Build history of the part. All positions in model axes, mm. Face numbers are marked on the shaded views. A direction names the side the tool comes from. Round coordinates to 2 decimals unless told otherwise and drop trailing zeros. Write each loop counter-clockwise with the first axis right and the second up, starting at its lowest first coordinate (ties: lowest second). Pieces come first, ordered by that corner, then holes. Notation, with made-up numbers: M -21.5,-37 L -2.5,-37 A27 cw -2.5,-20 Z; hole C 34,-14.75 d9. An arc over 180 degrees is marked long. Write item = value, one per line. Start each with the question number.
Q1. Tool access for the marked faces 4 and 5: list every direction of +Z, -Z, +X, -X, +Y, -Y with a clear straight run to the whole face (end or side of a thin tool).
Q2. Pull direction Y, two halves, no side cores. Call the marked faces 1, 2 and 3: released by +Y, released by -Y, zero draft, split by the parting line, or undercut.
Q3. Probe L1, parallel to X at y = 0.25, z = 2.75; L2, parallel to Z at x = 11.5, y = 0; L3, parallel to Z at x = -1, y = 0.75. List the from-to ranges inside material, lowest first.
Q4. Band-saw the part on A-A on x = 8.5. Write the cut outline in (y, z).
Q5. Drop flat-ended pins along their axis: P1, Ø1, axis at x = 6.5, z = 1.5, coming from the +Y side; P2, Ø1.5, axis at x = 1.5, z = 0.5, coming from the +Y side; P3, Ø0.8, axis at y = -1, z = -1.5, coming from the +X side; P4, Ø0.5, axis at y = -1.5, z = 1.5, coming from the +X side. Give the stop position or say it passes through.
Autodesk Inventor part; units mm, degrees
ref_plane "Work Plane1" through (10.35, 0, 0) normal (0, -0.6335, -0.7737) x (1, 0, 0)
ref_plane "YZ Plane" through (0, 0, 0) normal (1, 0, 0) x (0, 1, 0)
ref_plane "XZ Plane" through (0, 0, 0) normal (0, 1, 0) x (-1, 0, 0)
sketch "Szkic1" plane through (0, 0, 0) normal (0, 0, 1) x (1, 0, 0)
  line L0 (0.0003, 0) -> (20, 0)
  line L1 (20, 0) -> (20, 2)
  line L2 (20, 2) -> (0.7, 2)
  line L3 (0.7, 2) -> (0.2706, 1.8)
  line L4 (0.2706, 1.8) -> (0, 1.8)
  line L5 (0, 1.8) -> (0, 3.5)
  line L6 (0, 3.5) -> (-2.8, 3.5)
  line L7 (-2.8, 3.5) -> (-2.8, 1.975)
  line L8 (-2.8, 1.975) -> (-1.14, 1.975)
  line L9 (-1.14, 1.975) -> (0.0003, 0)
  line L10 (-7.36, 0) -> (24.56, 0)
  line L11 (0, -0.7) -> (0, 4.2)
  line L12 (0.7, 2) -> (0, 2) construction
  dimension "d1" = 19.3
  dimension "d2" = 0.4294
  dimension "d3" = 2.8
  dimension "d4" = 1.66
  dimension "d5" = 60
  dimension "d6" = 4
  dimension "d7" = 3.6
  dimension "d8" = 3.95
  dimension "d9" = 7
  dimension "d20" = 20
revolve "Bryła" add sketch "Szkic1" angle 360 about axis through (0.0003, 0, 0) along (1, 0, 0)
sketch "Szkic2" plane through (-2.8, 0, 0) normal (-1, 0, 0) x (0, 0, 1)
  line L0 (0, -4.9) -> (0, 4.9)
  line L1 (-4.9, 0) -> (4.9, 0)
  circle A0 centre (0, 0) radius 1.975 construction
  circle A1 centre (0, 0) radius 1.425 construction
  line L2 (0, 0) -> (1.7104, 0.9875) construction
  line L3 (0, 0) -> (0.9875, 1.7104) construction
  arc A2 (1.1195, 1.4173) -> (0.6677, 1.6781) centre (0.85, 1.4722) ccw
  arc A3 (1.1195, 1.4173) -> (1.7871, 0.2608) centre (2.1063, 1.2161) ccw
  arc A4 (1.7871, -0.2608) -> (1.7871, 0.2608) centre (1.7, 0) ccw
  arc A5 (1.7871, -0.2608) -> (1.1195, -1.4173) centre (2.1063, -1.2161) ccw
  arc A6 (-0.6677, 1.6781) -> (0.6677, 1.6781) centre (0, 2.4322) ccw
  arc A7 (-0.6677, 1.6781) -> (-1.1195, 1.4173) centre (-0.85, 1.4722) ccw
  arc A8 (-1.7871, 0.2608) -> (-1.1195, 1.4173) centre (-2.1063, 1.2161) ccw
  arc A9 (-1.7871, 0.2608) -> (-1.7871, -0.2608) centre (-1.7, 0) ccw
  arc A10 (-1.1195, -1.4173) -> (-1.7871, -0.2608) centre (-2.1063, -1.2161) ccw
  arc A11 (0.6677, -1.6781) -> (1.1195, -1.4173) centre (0.85, -1.4722) ccw
  arc A12 (0.6677, -1.6781) -> (-0.6677, -1.6781) centre (0, -2.4322) ccw
  arc A13 (-1.1195, -1.4173) -> (-0.6677, -1.6781) centre (-0.85, -1.4722) ccw
  circle A14 centre (0, 0) radius 1.975
  dimension "d34" = 30
  dimension "d35" = 60
  dimension "d36" = 2.85
  dimension "d37" = 3.95
  dimension "d38" = 0.275
extrude "Szczelina" add sketch "Szkic2" against normal blind 1.66 contours A14 A13 A12 L0 | L0 A12 A11 A14 | A14 A9 A10 A13 | A11 A5 A4 A14 | A14 A7 A8 A9 | A4 A3 A2 A14 | A6 A7 A14 L0 | L0 A14 A2 A6
fillet "Zaokrąglenie1" radius 0.2 1 edges at (-2.8, -3.5, 0)
thread "Gwint"
chamfer "Faza1" distance 0.2634 distance2 0.4295 1 edges at (20, -2, 0) measured on face at (20, 0.527, -0.2661)
ref_plane "Work Plane1" through (10.35, 0, 0) normal (0, -0.6335, -0.7737) x (1, 0, 0)
equation "\"d1\" = GEL"
equation "\"d2\" = GAL"
equation "\"d3\" = KOH"
equation "\"d4\" = INTI"
equation "\"d6\" = GD"
equation "\"d7\" = BDM"
equation "\"d8\" = SW"
equation "\"d9\" = KOD"
equation "\"d20\" = NLG"
equation "\"d36\" = E0"
equation "\"d37\" = SW"
equation "\"d38\" = -0.25 * E0 + 0.25 * SW"
equation "\"d11\" = INTI"
equation "\"d17\" = RR"
equation "\"d13\" = GEL"
equation "\"d15\" = -0.5 * SPD + 0.5 * GD"
equation "\"GD\" = NND"
equation "\"NLG\" = 20"
equation "\"GEL\" = 19.3"
equation "\"KOD\" = 7"
equation "\"KOH\" = 2.8"
equation "\"INTI\" = 1.66"
equation "\"GAL\" = 0.61345 * PTC"
equation "\"GUL\" = 0.61345 * PTC"
equation "\"BDM\" = 3.6"
equation "\"SW\" = 3.95"
equation "\"RR\" = 0.2"
equation "\"SPD\" = NND - 1.2269 * GAL"
equation "\"E0\" = 2.85"
equation "\"TOA\" = 30deg"
equation "\"GD1\" = THREADDIA - 1.2269 * PTC"
equation "\"THREADDIA\" = 4"
equation "\"PTC\" = 0.7"
equation "\"NND\" = 4"
equation "\"RRK\" = 0.29"
properties part number "NF E 25-111 - M4x20 Klasa właściwości 4.8" material "Stal, miękka"
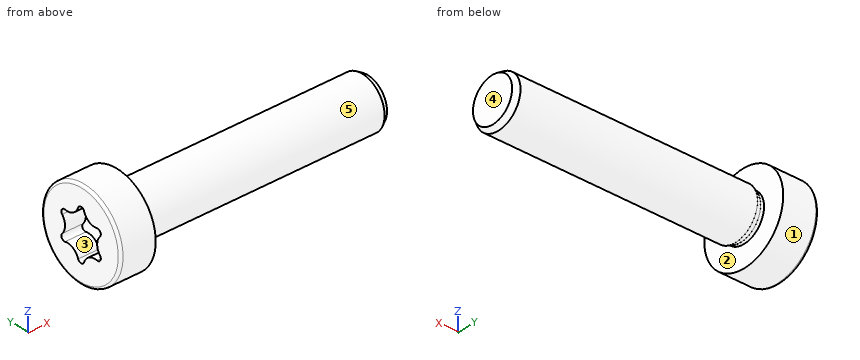
Conclusion:
q1.face_4 = +Z, -Z, +X, +Y, -Y
q1.face_5 = +X
q2.face_1 = split by the parting line
q2.face_2 = zero draft
q2.face_3 = undercut
q3.L1 = -2.8 to 0
q3.L2 = -2 to 2
q3.L3 = -3.42 to -1.56, 1.56 to 3.42
q4.outline = C 0,0 d4
q5.P1 = 1.73
q5.P2 = 2
q5.P3 = 20
q5.P4 = 19.78
